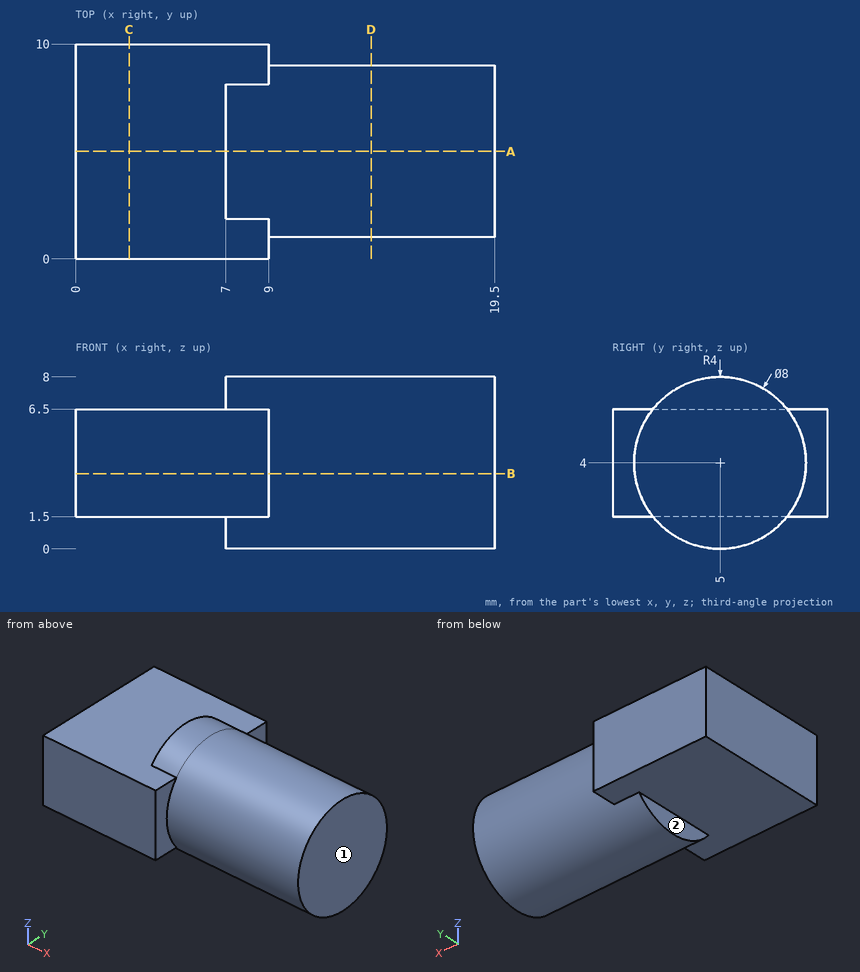
Can you work these out from the drawing? Everything is in mm from the part's minimum corner. A direction names the side the tool comes from. Give positions to 0.01 mm unless a question says otherwise; leave off trailing zeros. Loops run counter-clockwise (first coordinate to the right, second up) from the corner with the lowest first, then second, coordinate; pieces in that order, holes last. Notation, with made-up numbers: M 34,-12.75 L 54,-12.75 A13 ccw 54,0.25 Z; hole C 11,89.25 d2. An arc over 180 degrees is marked long. Put each result on its own line as item: value. Start each with the question number.
(1) I want a section at B-B on z = 3.5. Please give me the cut outline in (x, y).
(2) I want a section at D-D on x = 13.75. Please give me the cut outline in (y, z).
(3) Will these pins go through, and if not, where does the flat tip stop? pin 1 Ø4 at (x, z) = (14, 6) entering from +Y; pin 2 Ø2.5 at (x, y) = (4, 5.5) entering from +Z; pin 3 Ø3 at (x, y) = (11.5, 2.5) entering from -Z.
(4) I need wall thicknesses on line 1 along Z through (x, y) = (2.25, 4.5); line 2 along X through (y, z) = (4.75, 7.5); line 3 along X through (y, z) = (9.5, 4.5). Which ranges of each line are inside material? Lowest first, please. Write a range as [from, to].
(5) For the marked faces 1 and 2, which set-ups out of +Z, -Z, +X, -X, +Y, -Y let a thin tool reach every point of the face, with its end or its side?
(6) I want a section at A-A on y = 5. Please give me the cut outline in (x, z), then the cut area to 3 significant figures.
(7) I want a section at C-C on x = 2.5. Please give me the cut outline in (y, z).
Answer block:
1. outline: M 0,0 L 9,0 L 9,1.03 L 19.5,1.03 L 19.5,8.97 L 9,8.97 L 9,10 L 0,10 Z
2. outline: C 5,4 d8
3. pin 1: y = 9
3. pin 2: z = 6.5
3. pin 3: z = 0.13
4. line 1: [1.5, 6.5]
4. line 2: [7, 19.5]
4. line 3: [0, 9]
5. face 1: +Z, -Z, +X, +Y, -Y
5. face 2: -Z, -X, +Y, -Y
6. outline: M 0,1.5 L 7,1.5 L 7,0 L 19.5,0 L 19.5,8 L 7,8 L 7,6.5 L 0,6.5 Z
6. area: 135 mm^2
7. outline: M 0,1.5 L 10,1.5 L 10,6.5 L 0,6.5 Z
